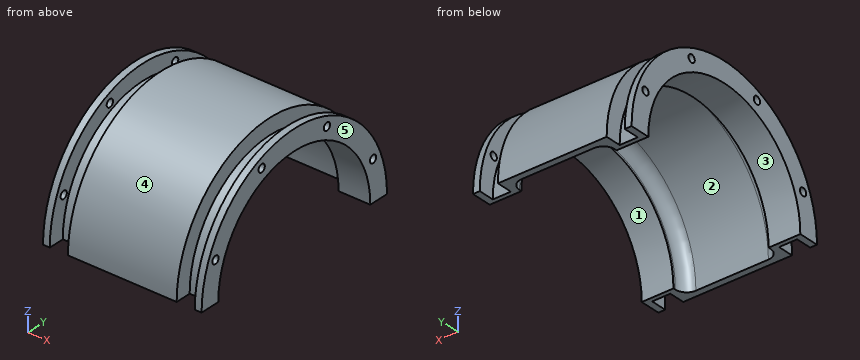
```python
from build123d import *

# Parameters (mm, degrees)
REVOLVE_1_ANGLE          = 180
HOLE_WIZARD_M3_1_D       = 3.4
HOLE_WIZARD_M3_1_DEPTH   = 3
PATTERN_CIRCULAR_1_COUNT = 4
PATTERN_CIRCULAR_1_ANGLE = 135
MIRROR_1_COPY_1_D        = 3.4
MIRROR_1_COPY_1_DEPTH    = 3
MIRROR_1_COPY_2_D        = 3.4
MIRROR_1_COPY_2_DEPTH    = 3
MIRROR_1_COPY_3_D        = 3.4
MIRROR_1_COPY_3_DEPTH    = 3
FILLET_1_R               = 5


with BuildPart() as part:
    # ｽｹｯﾁ1 → 回転1 (revolve)
    with BuildSketch(Plane.XY):
        Polygon((-35, 41), (-21, 41), (-21, 47), (21, 47), (21, 41), (35, 41), (35, 50), (32, 50), (32, 43), (24, 43), (24, 50), (-24, 50), (-24, 43), (-32, 43), (-32, 50), (-35, 50), align=None)
    revolve(axis=Axis((-50, 0, 0), (1, 0, 0)), revolution_arc=REVOLVE_1_ANGLE)

    # M3 すきま穴1
    with Locations(Plane.ZY.offset(35)):
        with Locations((17.603437889, -42.498458496)):
            hole_wizard_m3_1 = Hole(HOLE_WIZARD_M3_1_D / 2, depth=HOLE_WIZARD_M3_1_DEPTH)

    # 円形ﾊﾟﾀｰﾝ1: M3 すきま穴1 ×4 about axis
    pattern_circular_1_axis = Axis((0, 0, 0), (-1, 0, 0))
    for i in range(1, PATTERN_CIRCULAR_1_COUNT):
        add(hole_wizard_m3_1.rotate(pattern_circular_1_axis, i * PATTERN_CIRCULAR_1_ANGLE / (PATTERN_CIRCULAR_1_COUNT - 1)), mode=Mode.SUBTRACT)

    # ﾐﾗｰ1: M3 すきま穴1 across plane
    add(hole_wizard_m3_1.mirror(Plane(origin=(0, 0, 0), x_dir=(0, 0, 1), z_dir=(1, 0, 0))), mode=Mode.SUBTRACT)

    # ﾐﾗｰ1 copy 1
    with Locations(Plane(origin=(35, 0, 0), x_dir=(0, 0.7071067811865487, 0.7071067811865464), z_dir=(1, 0, 0))):
        with Locations((17.603437889, 42.498458496)):
            Hole(MIRROR_1_COPY_1_D / 2, depth=MIRROR_1_COPY_1_DEPTH)

    # ﾐﾗｰ1 copy 2
    with Locations(Plane.YZ.offset(35)):
        with Locations((17.603437889, 42.498458496)):
            Hole(MIRROR_1_COPY_2_D / 2, depth=MIRROR_1_COPY_2_DEPTH)

    # ﾐﾗｰ1 copy 3
    with Locations(Plane(origin=(35, 0, 0), x_dir=(0, 0.7071067811865441, -0.7071067811865509), z_dir=(1, 0, 0))):
        with Locations((17.603437889, 42.498458496)):
            Hole(MIRROR_1_COPY_3_D / 2, depth=MIRROR_1_COPY_3_DEPTH)

    # ﾌｨﾚｯﾄ1
    fillet_1_edges = [part.edges().sort_by_distance(p)[0] for p in [
        (21, 0, 47),
        (-21, 0, 47),
    ]]
    fillet(fillet_1_edges, radius=FILLET_1_R)


solid = part.part
```
CAD build for the part. Positions are in the model's coordinates, mm. Face numbers are marked on the shaded views. A direction names the side the tool comes from. Round coordinates to 2 decimals unless told otherwise and drop trailing zeros. Loops run counter-clockwise (first coordinate to the right, second up) from the corner with the lowest first, then second, coordinate; pieces in that order, holes last. Notation, with made-up numbers: M -33.75,-32.75 L 11.25,-32.75 A21 cw 11.25,-28.75 Z; hole C -9.5,-20.75 d5. An arc over 180 degrees is marked long. Use a Markdown table: item, result. Add a question column.
(1) Cut at A-A (y = 0). Give the cut face in (x, z), and give its area (3 significant figures).
(2) Cut at C-C (x = -4.5). Give the cut face in (y, z).
(3) Pull direction Y, two halves, no side cores. Call the marked faces 3, 4 and 5: +Y half, -Y half, draft (parallel to the pull), parting line (faces both ways), or undercut.
(4) Flat gauge pins, fed straight in: pin 1 (3 mm diameter, centred on x = -1.5, y = -20, fed in from -Z); pin 2 (2 mm diameter, centred on x = 20, z = 38, fed in from +Y); pin 3 (1.5 mm diameter, centred on x = -2, z = 32.5, fed in from +Y). Where does each tip first touch, or does it go through?
(5) Which spindle directions (+Z, -Z, +X, -X, +Y, -Y) get a long thin tool onto all of the face, cutting with end or side? Do the marked faces 1 and 2. Say none if no direction does.
(6) Cut at B-B (x = 25.5). Give the cut face in (y, z), and give its area (3 significant figures).
(7) Drill centre lines: line 1 (X direction, y = 8, z = 47); line 2 (X direction, y = -40.5, z = 20); line 3 (X direction, y = 39.5, z = 14.5). Where is each one in solid material? Low to high.
Geometry says:
| question | item | result |
|---|---|---|
| 1 | outline | M -35,41 L -21,41 L -21,42 A5 cw -16,47 L 16,47 A5 cw 21,42 L 21,41 L 35,41 L 35,50 L 32,50 L 32,43 L 24,43 L 24,50 L -24,50 L -24,43 L -32,43 L -32,50 L -35,50 Z |
| 1 | area | 277 mm² |
| 2 | outline | M -50,0 L -47,0 A47 cw 47,0 L 50,0 A50 ccw Z |
| 3 | face 3 | undercut |
| 3 | face 4 | parting line |
| 3 | face 5 | draft |
| 4 | pin 1 | stops at z = 41.79 |
| 4 | pin 2 | stops at y = 33.63 |
| 4 | pin 3 | stops at y = 38.63 |
| 5 | face 1 | -Z, +X, -X |
| 5 | face 2 | -Z |
| 6 | outline | M -43,0 L -41,0 A41 cw 41,0 L 43,0 A43 ccw Z |
| 6 | area | 264 mm² |
| 7 | line 1 | x = -35 to -32, -24 to 24, 32 to 35 |
| 7 | line 2 | x = -35 to -32, -24 to -19.87, 19.87 to 24, 32 to 35 |
| 7 | line 3 | x = -35 to -21, 21 to 35 |
